```python
from build123d import *

# Parameters (mm, degrees)
F0_W     = 6
F0_H     = 10
F1_DEPTH = 67.5
F0_R     = 10
F0_W_2   = 7
F0_W_3   = 37
F2_DEPTH = 37.5
F3_DEPTH = 3
F4_W     = 10
F4_H     = 55
F5_DEPTH = 90.001
F6_R     = 6
F7_DEPTH = 75.001


with BuildPart() as f1:
    # F0 (on Top) → F1 (new body, symmetric)
    with BuildSketch(Plane.XY):
        Polygon((0, 10), (0, 0), (90, 0), (90, 10), (53, 10), (47, 10), (40, 10), align=None)
        with Locations((50, 15)):
            Rectangle(F0_W, F0_H)
    extrude(amount=F1_DEPTH, both=True)

    # F0 (on Top) → F2 (join, symmetric)
    with BuildSketch(Plane.XY):
        with BuildLine():
            Line((0, 55), (0, 10))
            Line((0, 10), (40, 10))
            Line((40, 10), (40, 20))
            Line((40, 20), (40, 55))
            ThreePointArc((40, 55), (38.226001, 63.234858), (33.218712, 70.008853))
            ThreePointArc((33.218712, 70.008853), (11.765142, 73.226001), (0, 55))
        make_face()
        with Locations((20, 55)):
            Circle(F0_R, mode=Mode.SUBTRACT)
        with Locations((43.5, 15)):
            Rectangle(F0_W_2, F0_H)
        with Locations((71.5, 15)):
            Rectangle(F0_W_3, F0_H)
        with Locations((50, 15)):
            Rectangle(F0_W, F0_H)
    extrude(amount=F2_DEPTH, both=True)

    # F0 (on Top) → F3 (join, symmetric)
    with BuildSketch(Plane.XY):
        with BuildLine():
            Line((53, 20), (90, 20))
            Line((90, 20), (33.218712, 70.008853))
            ThreePointArc((33.218712, 70.008853), (38.226001, 63.234858), (40, 55))
            Line((40, 55), (40, 20))
            Line((40, 20), (47, 20))
            Line((47, 20), (53, 20))
        make_face()
    extrude(amount=F3_DEPTH, both=True)

    # F4 (on face) → F5 (cut, through all)
    with BuildSketch(Plane.YZ.offset(90)):
        Polygon((10, 67.5), (20, 37.5), (20, 67.5), align=None)
        Polygon((20, -67.5), (20, -37.5), (10, -67.5), align=None)
        with Locations((5, 0)):
            Rectangle(F4_W, F4_H)
    extrude(amount=-F5_DEPTH, mode=Mode.SUBTRACT)

    # F6 (on face) → F7 (cut, through all)
    with BuildSketch(Plane.XZ):
        with Locations((70, 52.5)):
            Circle(F6_R)
        with Locations((20, 52.5)):
            Circle(F6_R)
        with Locations((70, -52.5)):
            Circle(F6_R)
        with Locations((20, -52.5)):
            Circle(F6_R)
    extrude(amount=-F7_DEPTH, mode=Mode.SUBTRACT)


solid = f1.part
```
The model under review builds one solid part; all positions refer to its coordinate system, in mm. A direction names the side the tool comes from. Give positions to 0.01 mm unless a question says otherwise; leave off trailing zeros. Write each loop counter-clockwise with the first axis right and the second up, starting at its lowest first coordinate (ties: lowest second). Pieces come first, ordered by that corner, then holes.
(1) Consider section C-C, the plane y = 52.5. Give the boundary of the cut face in (x, z).
(2) For P1, Ø10.5, axis at y = 43.5, z = 22.5, coming from the +X side; P2, Ø12, axis at x = 36.5, y = 20.5, coming from the -Z side; P3, Ø8, axis at x = 58.5, z = 13.5, coming from the +Y side, all flat-tipped, find the tip position at first contact; note any pin that passes through.
(3) Tool access review of faces 1 (the flat face through (46, 5, 27.5)), 2 (the flat face through (23, 36, -37.5)), 3 (the flat face through (29, 10, 53)), 4 (the flat face through (55, 34, 3)), 5 (the flat face through (53, 14, -49)): name each direction out of +Z, -Z, +X, -X, +Y, -Y from which nothing blocks a thin tool from reaching the whole face with its end or side.
(4) Consider section A-A, the plane z = -52.5. Give the boundary of the cut face in (x, y), and give its area (3 significant figures).
(5) Consider section D-D, the plane z = -16. Give the boundary of the cut face in (x, y).
(6) Consider section B-B, the plane x = 20. Give the boundary of the cut face in (y, z).
(7) To check wall thickness, follow L1, parallel to Z at x = 70, y = 6.75; L2, parallel to X at y = 6, z = 52; L3, parallel to Y at x = 20, z = -11. State the ranges of each line that lie inside material, in increasing order.
(8) The part is to be moulded in two halves that separate along Z. For faces 6 (the flat face through (23, 36, 37.5)), 7 (the cylindrical face through (64.006, 4.93, 52.764)), 8 (the flat face through (47, 13, 46)), say which applies: released by +Z, released by -Z, zero draft, split by the parting line, or undercut.
Returned:
1. outline: (0, -37.5) - (10.32, -37.5) - (10.32, 37.5) - (0, 37.5) - close; (29.68, -37.5) - (40, -37.5) - (40, -3) - (53.1, -3) - (53.1, 3) - (40, 3) - (40, 37.5) - (29.68, 37.5) - close
2. P1: stops at x = 40
2. P2: stops at z = -37.5
2. P3: stops at y = 20
3. face 1: +X, -X, -Y
3. face 2: -Z, -X, +Y
3. face 3: +Z, -X, +Y
3. face 4: +Z, +X, +Y
3. face 5: -Z, +X, +Y
4. outline: (0, 0) - (14, 0) - (14, 10) - (0, 10) - close; (26, 0) - (64, 0) - (64, 10) - (53, 10) - (53, 15) - (47, 15) - (47, 10) - (26, 10) - close; (76, 0) - (90, 0) - (90, 10) - (76, 10) - close
4. area: 690 mm2
5. outline: (0, 10) - (90, 10) - (90, 20) - (40, 20) - (40, 55) arc R20 ccw to (33.22, 70.01) arc R20 ccw to (0, 55) - close; hole circle Ø20 at (20, 55)
6. outline: (0, -67.5) - (10, -67.5) - (10, -58.5) - (0, -58.5) - close; (0, -46.5) - (10, -46.5) - (10, -37.5) - (45, -37.5) - (45, 37.5) - (10, 37.5) - (10, 46.5) - (0, 46.5) - (0, 27.5) - (10, 27.5) - (10, -27.5) - (0, -27.5) - close; (0, 58.5) - (10, 58.5) - (10, 67.5) - (0, 67.5) - close; (65, -37.5) - (75, -37.5) - (75, 37.5) - (65, 37.5) - close
7. L1: z = -67.5 to -58.5, -46.5 to -27.5, 27.5 to 46.5, 58.5 to 67.5
7. L2: x = 0 to 14.02, 25.98 to 64.02, 75.98 to 90
7. L3: y = 10 to 45, 65 to 75
8. face 6: released by +Z
8. face 7: undercut
8. face 8: zero draft
